Geometry: see drawing. Coordinates: mm, zero at the bounding-box minimum. Round coordinates to 2 decimals unless told otherwise and drop trailing zeros. Order: outer loops, then holes, each group sorted by start corner. A loop starts at its lowest first (then second) coordinate and runs counter-clockwise, first axis right, second up. Notation, with made-up numbers: (15.25, -13) -> (24.25, -13) arc R29 cw to (24.25, 21) -> close; hole circle Ø1 at (-29.75, -13.5). An arc over 180 degrees is marked (long way). Answer as CSV lines item,"result". Start each with the question number.
(1) Section query A-A (y = 7). Output: boundary loops of the cut face in (x, z).
(2) Section query B-B (z = 9.5). Count the separate pieces of the cut face and the enclosed holes in it, plus the area to 3 significant figures.
(3) Line query: line 1 along X through (y, z) = (13.25, 10); line 2 along Z through (x, y) = (9, 5.5). Output: solid intervals per line, ascending. Write a range as from..to.
(4) Contact query for flat-ended pins moving along their axis: P1, Ø2, axis at x = 10, z = 3.5, coming from the +Y side; P2, Ø3, axis at x = 3.5, z = 10, coming from the +Y side; P3, Ø5, axis at y = 4, z = 16, coming from the +X side; P4, Ø1, axis at x = 13.5, y = 13, coming from the +Z side. Output: stop coordinate, or through.
(5) Pull-direction query (Z, two-part tool) for the marked faces 1, 2 and 3; classes: +Z half, -Z half, draft (parallel to the pull), parting line (faces both ways), or undercut.
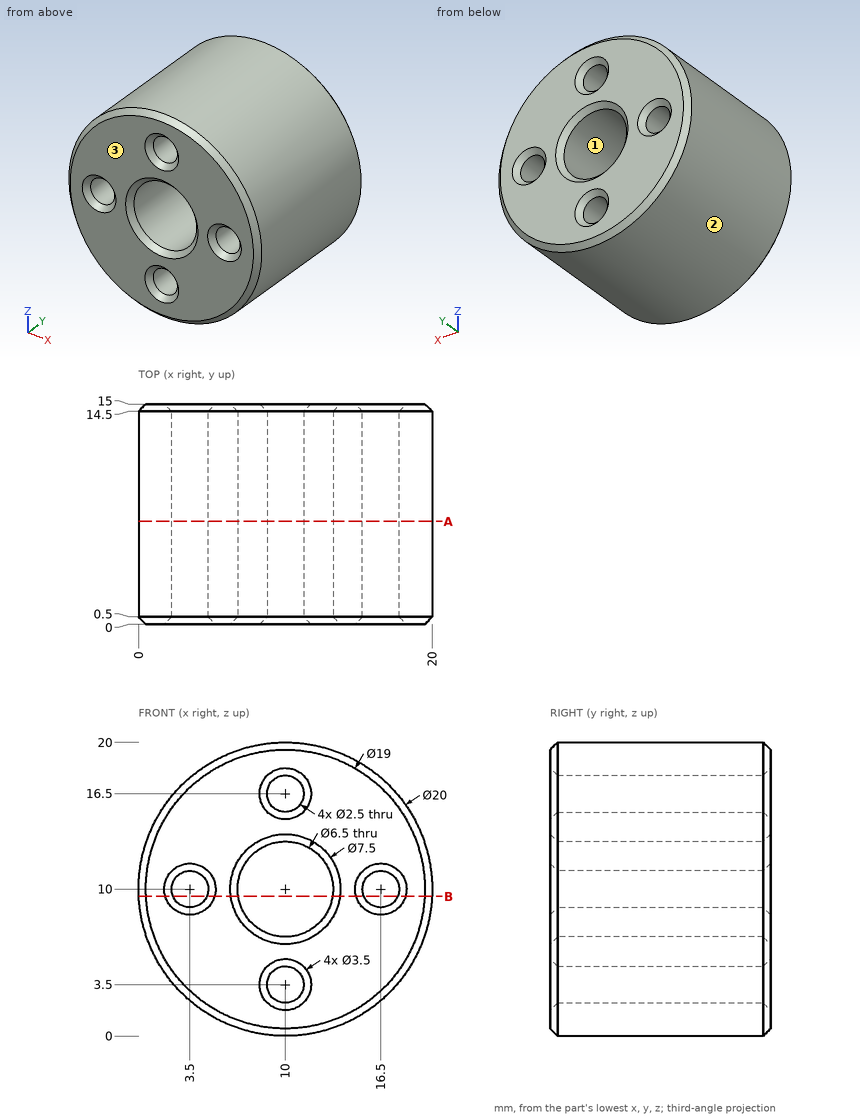
Answer block:
1,outline,"circle Ø20 at (10, 10); hole circle Ø2.5 at (3.5, 10); hole circle Ø6.5 at (10, 10); hole circle Ø2.5 at (10, 3.5); hole circle Ø2.5 at (10, 16.5); hole circle Ø2.5 at (16.5, 10)"
2,separate pieces,"4"
2,enclosed holes,"0"
2,area,"132 mm2"
3,line 1,"0..2.25, 4.75..6.75, 13.25..15.25, 17.75..20"
3,line 2,"0.05..2.75, 4.25..6.91, 13.09..15.75, 17.25..19.95"
4,P1,"through"
4,P2,"y = 14.75"
4,P3,"x = 19.37"
4,P4,"z = 19.54"
5,face 1,"undercut"
5,face 2,"parting line"
5,face 3,"draft"
